Here's how the part is built. I have some questions about the finished solid (model axes, mm). Face numbers are marked on the shaded views. A direction names the side the tool comes from. Coordinates: 2 decimals unless noted, no trailing zeros. Write each loop counter-clockwise with the first axis right and the second up, starting at its lowest first coordinate (ties: lowest second). Pieces come first, ordered by that corner, then holes. Notation, with made-up numbers: M 42,-9 L 79,-9 A13 ccw 79,-2 Z; hole C -25,54 d8. An arc over 180 degrees is marked long. Use one line per item in the form item = value. Start each with the question number.
1. I want a section at C-C, the plane x = 0. List the corners of the cut face in (y, z) for me.
2. On a 3-axis mill with a long thin cutter (end or side, diameter ignored), from which of +Z, -Z, +X, -X, +Y, -Y can I reach the whole of each face in a straight line? I mean the marked faces 1 and 2. Say none if no direction works.
3. Please list where these lines run through material, in increasing order: line 1 along X through (y, z) = (3.7, -15.5); line 2 along Z through (x, y) = (0, 1.15); line 3 along Z through (x, y) = (16, 3.65). Write a range as [from, to].
4. I want a section at A-A, the plane x = 15.5. List the corners of the cut face in (y, z) for me, plus the area to 3 significant figures.
5. I want a section at D-D, the plane z = 0. List the corners of the cut face in (x, y) for me.
6. I want a section at B-B, the plane z = 15.5. List the corners of the cut face in (x, y) for me.
from build123d import *

# Parameters (mm, degrees)
SKETCH1_W           = 52
SKETCH1_H           = 52
BOSS_EXTRUDE1_DEPTH = 5
SKETCH1_5_R         = 1.5
CUT_EXTRUDE2_DEPTH  = 13
SKETCH1_8_R         = 10
CUT_EXTRUDE5_DEPTH  = 3
SKETCH1_9_R         = 3
CUT_EXTRUDE6_DEPTH  = 24
SKETCH1_10_R        = 1.5
CUT_EXTRUDE7_DEPTH  = 24


with BuildPart() as part:
    # Sketch1 → Boss-Extrude1 (new body)
    with BuildSketch(Plane(origin=(0, 0, 0), x_dir=(1, 0, 0), z_dir=(0, 1, 0))):
        Rectangle(SKETCH1_W, SKETCH1_H)
    extrude(amount=BOSS_EXTRUDE1_DEPTH)

    # Sketch1<5> → Cut-Extrude2 (cut)
    with BuildSketch(Plane(origin=(0, 0, 0), x_dir=(1, 0, 0), z_dir=(0, 1, 0))):
        with Locations((22.627416998, 22.627416998)):
            Circle(SKETCH1_5_R)
        with Locations((22.627416998, -22.627416998)):
            Circle(SKETCH1_5_R)
        with Locations((-22.627416998, 22.627416998)):
            Circle(SKETCH1_5_R)
        with Locations((-22.627416998, -22.627416998)):
            Circle(SKETCH1_5_R)
        with Locations((15.5, -15.5)):
            Circle(SKETCH1_5_R)
        with Locations((-15.5, 15.5)):
            Circle(SKETCH1_5_R)
    extrude(amount=CUT_EXTRUDE2_DEPTH, mode=Mode.SUBTRACT)

    # Sketch1<8> → Cut-Extrude5 (cut)
    with BuildSketch(Plane(origin=(0, 0, 0), x_dir=(1, 0, 0), z_dir=(0, 1, 0))):
        Circle(SKETCH1_8_R)
    extrude(amount=CUT_EXTRUDE5_DEPTH, mode=Mode.SUBTRACT)

    # Sketch1<9> → Cut-Extrude6 (cut)
    with BuildSketch(Plane(origin=(0, 0, 0), x_dir=(1, 0, 0), z_dir=(0, 1, 0))):
        Circle(SKETCH1_9_R)
    extrude(amount=CUT_EXTRUDE6_DEPTH, mode=Mode.SUBTRACT)

    # Sketch1<10> → Cut-Extrude7 (cut)
    with BuildSketch(Plane(origin=(0, 0, 0), x_dir=(1, 0, 0), z_dir=(0, 1, 0))):
        with Locations((15.5, 15.5)):
            Circle(SKETCH1_10_R)
        with Locations((-15.5, -15.5)):
            Circle(SKETCH1_10_R)
    extrude(amount=CUT_EXTRUDE7_DEPTH, mode=Mode.SUBTRACT)


solid = part.part
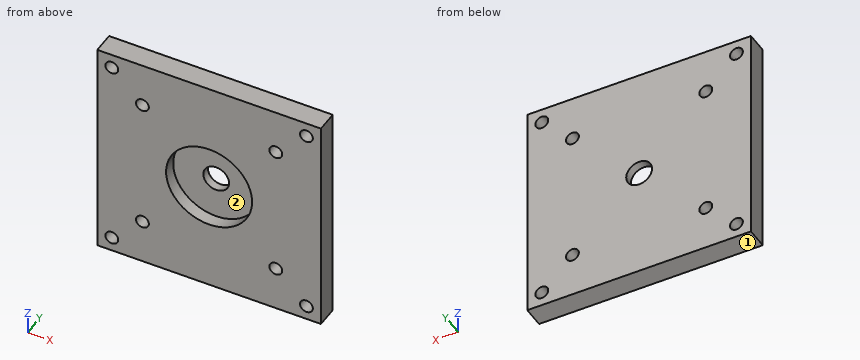
Answer list:
q1.outline = M 0,-26 L 5,-26 L 5,-3 L 3,-3 L 3,-10 L 0,-10 Z; M 0,10 L 3,10 L 3,3 L 5,3 L 5,26 L 0,26 Z
q2.face_1 = -Z, +X, -X, +Y, -Y
q2.face_2 = -Y
q3.line_1 = [-26, -17], [-14, 14], [17, 26]
q3.line_2 = [-26, -10], [10, 26]
q3.line_3 = [-26, -16.91], [-14.09, 14.09], [16.91, 26]
q4.outline = M 0,-26 L 5,-26 L 5,-17 L 0,-17 Z; M 0,-14 L 5,-14 L 5,14 L 0,14 Z; M 0,17 L 5,17 L 5,26 L 0,26 Z
q4.area = 230 mm²
q5.outline = M -26,0 L -10,0 L -10,3 L -3,3 L -3,5 L -26,5 Z; M 3,3 L 10,3 L 10,0 L 26,0 L 26,5 L 3,5 Z
q6.outline = M -26,0 L -17,0 L -17,5 L -26,5 Z; M -14,0 L 14,0 L 14,5 L -14,5 Z; M 17,0 L 26,0 L 26,5 L 17,5 Z
